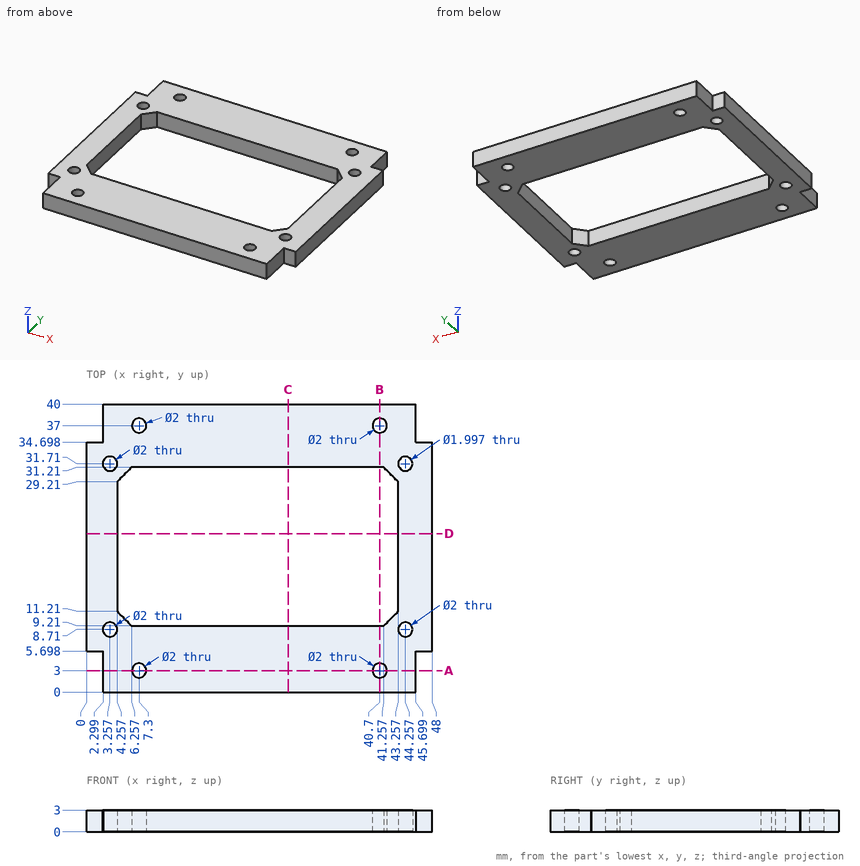
Geometry: see drawing. Coordinates: mm, zero at the bounding-box minimum. Coordinates: 2 decimals unless noted, no trailing zeros. Loops run counter-clockwise (first coordinate to the right, second up) from the corner with the lowest first, then second, coordinate; pieces in that order, holes last. Notation, with made-up numbers: M -22.5,-14 L 36.5,-14 A15 cw 36.5,3 Z; hole C 84,63 d3. An arc over 180 degrees is marked long. Put each result on its own line as item: value. Start each with the question number.
1) Cut plane C-C on x = 28. Return the cut outline in (y, z).
2) Contact query for flat-ended pins moving along their axis: pin 1 Ø1.8 at (x, z) = (47, 2) entering from +Y; pin 2 Ø1 at (x, y) = (30.5, 29) entering from -Z; pin 3 Ø1.5 at (y, z) = (3, 1) entering from +X; pin 4 Ø10 at (x, y) = (6.5, 13) entering from +Z. Output: stop coordinate, or through.
3) Ray query, L1, parallel to Y at x = 7.3, z = 0.9; L2, parallel to Y at x = 30, z = 1.65; L3, parallel to X at y = 19.5, z = 1.7. Return the intervals inside material, ascending. Write a range as from..to.
4) Cut plane B-B on x = 40.7. Return the cut outline in (y, z).
5) Cut plane A-A on y = 3. Return the cut outline in (x, z), then the cut area to 3 significant figures.
6) Cut plane D-D on y = 22. Return the cut outline in (x, z).
The answers:
1. outline: M 0,0 L 9.21,0 L 9.21,3 L 0,3 Z; M 31.21,0 L 40,0 L 40,3 L 31.21,3 Z
2. pin 1: stops at y = 34.7
2. pin 2: passes through
2. pin 3: stops at x = 45.7
2. pin 4: stops at z = 3
3. L1: y = 0..2, 4..9.21, 31.21..36, 38..40
3. L2: y = 0..9.21, 31.21..40
3. L3: x = 0..4.26, 43.26..48
4. outline: M 0,0 L 2,0 L 2,3 L 0,3 Z; M 4,0 L 9.21,0 L 9.21,3 L 4,3 Z; M 31.21,0 L 36,0 L 36,3 L 31.21,3 Z; M 38,0 L 40,0 L 40,3 L 38,3 Z
5. outline: M 2.3,0 L 6.3,0 L 6.3,3 L 2.3,3 Z; M 8.3,0 L 39.7,0 L 39.7,3 L 8.3,3 Z; M 41.7,0 L 45.7,0 L 45.7,3 L 41.7,3 Z
5. area: 118 mm²
6. outline: M 0,0 L 4.26,0 L 4.26,3 L 0,3 Z; M 43.26,0 L 48,0 L 48,3 L 43.26,3 Z
